Work out the finished part from the listing and answer in its coordinate system (mm). Face numbers are marked on the shaded views. A direction names the side the tool comes from. Give positions to 0.01 mm unless a question says otherwise; leave off trailing zeros. Order: outer loops, then holes, each group sorted by start corner. A loop starts at its lowest first (then second) coordinate and runs counter-clockwise, first axis right, second up. Notation, with made-up numbers: (34, 12) - (44, 12) arc R21 cw to (44, 43) - close; hole circle Ø3 at (19.5, -20). An arc over 180 degrees is marked (long way). Put each result on its own line as item: value.
Autodesk Inventor part; units mm, degrees
ref_plane "YZ Plane" through (0, 0, 0) normal (1, 0, 0) x (0, 1, 0)
ref_plane "XZ Plane" through (0, 0, 0) normal (0, 1, 0) x (-1, 0, 0)
ref_plane "XY Plane" through (0, 0, 0) normal (0, 0, 1) x (1, 0, 0)
sketch "스케치1" plane through (0, 0, 0) normal (0, 0, 1) x (1, 0, 0)
  line L0 (0, 0) -> (12, 0)
  line L1 (12, 0) -> (12, 20)
  line L2 (12, 20) -> (0, 20)
  line L3 (0, 20) -> (0, 0)
  dimension "d0" = 12
  dimension "d1" = 20
extrude "돌출1" add sketch "스케치1" along normal blind 3
sketch "스케치2" plane through (0, 0, 3) normal (0, 0, 1) x (1, 0, 0)
  line L0 (0, 20) -> (0, 0)
  line L1 (0, 0) -> (12, 0)
  line L2 (12, 0) -> (12, 20)
  line L3 (12, 20) -> (0, 20)
  line L4 (2, 20) -> (2, 0)
  line L5 (10, 20) -> (10, 0)
  line L6 (2, 2) -> (10, 2)
  dimension "d4" = 2
  dimension "d5" = 2
  dimension "d6" = 2
extrude "돌출2" add sketch "스케치2" along normal blind 12 contours L3 L4 L1 L0 | L4 L6 L5 L1 | L3 L2 L1 L5
sketch "스케치3" plane through (0, 0, 0) normal (0, 0, -1) x (-1, 0, 0)
  line L0 (0, 0) -> (-12, 0)
  circle A0 centre (-6, 5) radius 2.45
  circle A1 centre (-6, 15) radius 2.45
  point P0 (-6, 0)
  point P1 (-6, 0)
  dimension "d9" = 5
  dimension "d10" = 10
  dimension "d11" = 4.9
  dimension "d12" = 4.9
extrude "돌출3" cut sketch "스케치3" against normal blind 3
fillet "모깎기1" radius 2 2 edges at (12, 0, 7.5) (0, 0, 7.5)
properties part number "_3D 인쇄"
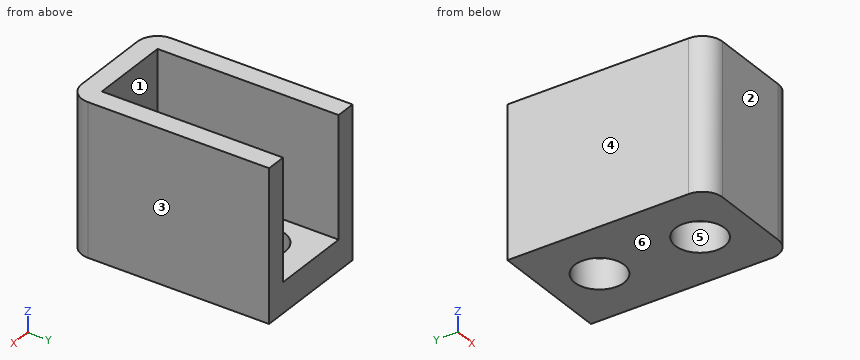
(1) Determine the mould class of the marked faces 3, 4, 5 and 6 for opening direction X: pulls with the +X half, pulls with the -X half, needs draft (parallel to the pull), parting line crosses it, or undercut.
Geometry check:
face 3: pulls with the +X half
face 4: pulls with the -X half
face 5: undercut
face 6: needs draft
(2) Given pin 1 (3 mm diameter, centred on x = 6, y = 5, fed in from +Z), flat-ended and moving along its own axis, determine where the tip first touches the part or whether it passes through.
Geometry check:
pin 1: passes through
(3) Section D-D, the plane z = 3.5 is taken. Write down the section's boundary in (x, y), then the cut area to 3 significant figures.
Geometry check:
outline: (0, 2) arc R2 ccw to (2, 0) - (10, 0) arc R2 ccw to (12, 2) - (12, 20) - (10, 20) - (10, 2) - (2, 2) - (2, 20) - (0, 20) - close
area: 94.3 mm²
(4) Section A-A, the plane x = 6 is taken. Write down the section's boundary in (y, z), then the cut area to 3 significant figures.
Geometry check:
outline: (0, 0) - (2.55, 0) - (2.55, 3) - (2, 3) - (2, 15) - (0, 15) - close; (7.45, 0) - (12.55, 0) - (12.55, 3) - (7.45, 3) - close; (17.45, 0) - (20, 0) - (20, 3) - (17.45, 3) - close
area: 54.6 mm²
(5) Section B-B, the plane z = 1.75 is taken. Write down the section's boundary in (x, y).
Geometry check:
outline: (0, 2) arc R2 ccw to (2, 0) - (10, 0) arc R2 ccw to (12, 2) - (12, 20) - (0, 20) - close; hole circle Ø4.9 at (6, 5); hole circle Ø4.9 at (6, 15)
(6) Straight lines are drawn through the part: line 1 (Y direction, x = 6, z = 1.5); line 2 (X direction, y = 3.5, z = 4.75); line 3 (Y direction, x = 8, z = 1). For each, find the intervals that lie inside material, in ascending order.
Geometry check:
line 1: y = 0 to 2.55, 7.45 to 12.55, 17.45 to 20
line 2: x = 0 to 2, 10 to 12
line 3: y = 0 to 3.58, 6.42 to 13.58, 16.42 to 20
(7) Section C-C, the plane y = 14.75 is taken. Write down the section's boundary in (x, z).
Geometry check:
outline: (0, 0) - (3.56, 0) - (3.56, 3) - (2, 3) - (2, 15) - (0, 15) - close; (8.44, 0) - (12, 0) - (12, 15) - (10, 15) - (10, 3) - (8.44, 3) - close
(8) A tool of negligible diameter and unlimited length cuts with its end or side. For the marked faces 1 and 2, from which of +Z, -Z, +X, -X, +Y, -Y can it reach the whole face along a straight path? Write none if from no direction.
Geometry check:
face 1: +Z, +Y
face 2: +Z, -Z, +X, -X, -Y
